For this review, take the finished solid that the model builds, in its own axes (mm). Give positions to 0.01 mm unless a question says otherwise; leave off trailing zeros. Loops run counter-clockwise (first coordinate to the right, second up) from the corner with the lowest first, then second, coordinate; pieces in that order, holes last. Notation, with made-up numbers: (54.25, -37.75) - (64.25, -37.75) arc R15 cw to (64.25, -11.75) - close; hole circle Ø6 at (60.5, -39.75). An arc over 180 degrees is marked (long way). Answer in a Markdown table with one row per item.
Autodesk Inventor part; units mm, degrees
ref_plane "YZ Plane" through (0, 0, 0) normal (1, 0, 0) x (0, 1, 0)
ref_plane "XZ Plane" through (0, 0, 0) normal (0, 1, 0) x (-1, 0, 0)
ref_plane "XY Plane" through (0, 0, 0) normal (0, 0, 1) x (1, 0, 0)
sketch "Sketch1" plane through (0, 0, 0) normal (0, 0, 1) x (1, 0, 0)
  line L0 (0, 0) -> (35, 0)
  line L1 (35, 0) -> (35, 420)
  line L2 (35, 420) -> (0, 420)
  line L3 (0, 420) -> (0, 0)
  dimension "d0" = 35
  dimension "d1" = 420
extrude "Extrusion1" add sketch "Sketch1" along normal blind 5
sketch "Sketch2" plane through (35, 0, 0) normal (1, 0, 0) x (0, 0, -1)
  circle A0 centre (-2.5, 410) radius 1
  circle A1 centre (-2.5, 210) radius 1
  circle A2 centre (-2.5, 10) radius 1
  line L0 (-5, 0) -> (-5, 420)
  line L1 (0, 420) -> (-5, 420)
  point P0 (0, 0)
  dimension "d4" = 2
  dimension "d5" = 2
  dimension "d6" = 2
  dimension "d7" = 2.5
  dimension "d8" = 2.5
  dimension "d9" = 2.5
  dimension "d10" = 10
  dimension "d11" = 210
  dimension "d12" = 410
extrude "Extrusion2" cut sketch "Sketch2" against normal blind 5
sketch "Sketch3" plane through (0, 0, 0) normal (-1, 0, 0) x (0, 0, 1)
  circle A0 centre (2.5, 10) radius 1
  circle A1 centre (2.5, 210) radius 1
  circle A2 centre (2.5, 410) radius 1
  line L0 (0, 420) -> (0, 0)
  line L1 (0, 420) -> (5, 420)
  dimension "d15" = 2
  dimension "d16" = 2.5
  dimension "d17" = 10
  dimension "d18" = 2
  dimension "d19" = 2.5
  dimension "d20" = 210
  dimension "d21" = 2
  dimension "d22" = 2.5
  dimension "d23" = 410
extrude "Extrusion3" cut sketch "Sketch3" against normal blind 5
sketch "Skizze4" plane through (0, 0, 5) normal (0, 0, 1) x (1, 0, 0)
  circle A0 centre (17.5, 320) radius 5
  circle A1 centre (17.5, 390) radius 5
  line L0 (0, 420) -> (0, 0)
  line L1 (0, 0) -> (35, 0)
  line L2 (35, 420) -> (0, 420)
  line L3 (17.5, 420) -> (17.5, 320) construction
  dimension "d26" = 17.5
  dimension "d27" = 17.5
  dimension "d29" = 70
  dimension "d32" = 30
  dimension "d33" = 10
extrude "Extrusion4" cut sketch "Skizze4" against normal blind 35
equation "\"d29\" = VerticalDistance"
equation "\"d30\" = d28"
properties part number "Side plate profile" material "Acetalharz, Weiß"
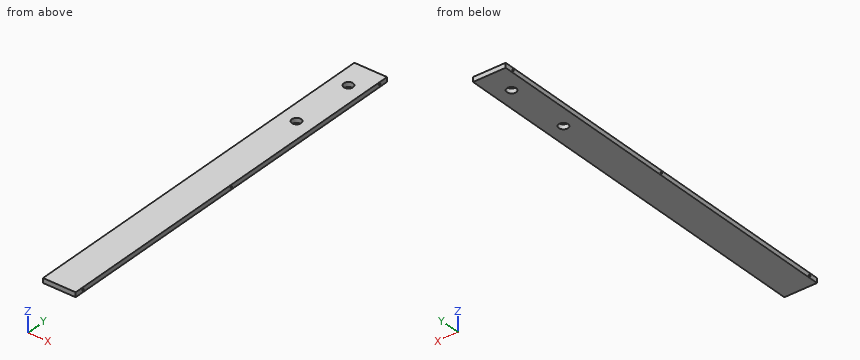
1. Clearance check with flat-ended pins moving along their axes: pin 1 (1.2 mm diameter, centred on y = 210, z = 2.5, fed in from -X); pin 2 (1.6 mm diameter, centred on y = 410, z = 2.5, fed in from +X). State where each tip first meets the part, or that it passes through.
Values:
| item | result |
|---|---|
| pin 1 | stops at x = 5 |
| pin 2 | stops at x = 30 |
2. We need section A-A, the plane y = 390. Give the boundary of the cut face in (x, z).
Values:
| item | result |
|---|---|
| outline | (0, 0) - (12.5, 0) - (12.5, 5) - (0, 5) - close; (22.5, 0) - (35, 0) - (35, 5) - (22.5, 5) - close |
3. Wall thickness on line 1 (Y direction, x = 1.2, z = 2.5); line 2 (Y direction, x = 17.5, z = 3.05); line 3 (X direction, y = 390, z = 3.2): over which ranges is each line inside the solid? List them lowest first. Write a range as [from, to].
Values:
| item | result |
|---|---|
| line 1 | y = [0, 9], [11, 209], [211, 409], [411, 420] |
| line 2 | y = [0, 315], [325, 385], [395, 420] |
| line 3 | x = [0, 12.5], [22.5, 35] |
